Geometry: final body of the model. Coordinates: model frame, mm. A direction names the side the tool comes from. Coordinates: 2 decimals unless noted, no trailing zeros. Order: outer loops, then holes, each group sorted by start corner. A loop starts at its lowest first (then second) coordinate and runs counter-clockwise, first axis right, second up. Notation, with made-up numbers: M 60,71 L 69,71 A13 cw 69,82 Z; hole C -5,64.5 d9. An arc over 180 degrees is marked long. One line per question, with ' | ' between items.
from build123d import *

# Parameters (mm, degrees)
SKETCH1_W                    = 31.75
SKETCH1_H                    = 63.5
SKETCH1_W_2                  = 25.4
SKETCH1_H_2                  = 57.15
BOSS_EXTRUDE1_DEPTH          = 720.4964
CUT_EXTRUDE1_REACH           = 725.554
F_10_0_1935_DIAMETER_HOLE1_D = 4.9149
SKETCH3_R                    = 9.525
CUT_EXTRUDE2_DEPTH           = 3.175


with BuildPart() as part:
    # Sketch1 → Boss-Extrude1 (new body)
    with BuildSketch(Plane.XY):
        with Locations((3.710272719, -29.23968021)):
            Rectangle(SKETCH1_W, SKETCH1_H)
        with Locations((3.710272719, -29.23968021)):
            Rectangle(SKETCH1_W_2, SKETCH1_H_2, mode=Mode.SUBTRACT)
    extrude(amount=BOSS_EXTRUDE1_DEPTH)

    # Cut-Extrude1: up to this face of the body (flat: up to its plane)
    cut_extrude1_end = Plane(part.part.faces().sort_by_distance((3.710272719, -60.98968021, 360.2482))[0])
    # Sketch2 → Cut-Extrude1 (cut, up to the picked face)
    with BuildSketch(Plane(origin=(0, 2.51031979, 0), x_dir=(1, 0, 0), z_dir=(0, 1, 0)), mode=Mode.PRIVATE) as cut_extrude1_sk1:
        Polygon((-12.164727281, -31.75), (13.235272719, 0), (-12.164727281, 0), align=None)
    cut_extrude1_tool1 = split(extrude(cut_extrude1_sk1.sketch, amount=-CUT_EXTRUDE1_REACH, mode=Mode.PRIVATE), bisect_by=cut_extrude1_end, keep=Keep.BOTH, mode=Mode.PRIVATE)
    # Sketch2 → Cut-Extrude1 (cut, up to the picked face)
    with BuildSketch(Plane(origin=(0, 2.51031979, 0), x_dir=(1, 0, 0), z_dir=(0, 1, 0)), mode=Mode.PRIVATE) as cut_extrude1_sk2:
        Polygon((13.235272719, -720.4964), (-12.164727281, -688.7464), (-12.164727281, -720.4964), align=None)
    cut_extrude1_tool2 = split(extrude(cut_extrude1_sk2.sketch, amount=-CUT_EXTRUDE1_REACH, mode=Mode.PRIVATE), bisect_by=cut_extrude1_end, keep=Keep.BOTH, mode=Mode.PRIVATE)
    add(cut_extrude1_tool1.solids().sort_by(Axis((-3.698061, 2.51032, 10.583333), (0, -1, 0)))[0], mode=Mode.SUBTRACT)
    add(cut_extrude1_tool2.solids().sort_by(Axis((-3.698061, 2.51032, 709.913067), (0, -1, 0)))[0], mode=Mode.SUBTRACT)

    # #10 (0.1935) Diameter Hole1 (through all)
    with Locations(Plane(origin=(16.410272719, -10.18968021, 15.875), x_dir=(0, -1, 0), z_dir=(-1, 0, 0))):
        with Locations((0, 0), (38.1, 0), (0, 688.7464), (38.1, 688.7464)):
            Hole(F_10_0_1935_DIAMETER_HOLE1_D / 2)

    # Sketch3 → Cut-Extrude2 (cut)
    with BuildSketch(Plane.ZY.offset(-16.410272719)):
        with Locations(Location((15.875, -29.23968021, 0), (0, 0, 270))):
            Circle(SKETCH3_R)
        with Locations(Location((704.6214, -29.23968021, 0), (0, 0, 270))):
            Circle(SKETCH3_R)
    extrude(amount=-CUT_EXTRUDE2_DEPTH, mode=Mode.SUBTRACT)


solid = part.part
1. Section C-C, the plane x = 7.5. Output: boundary loops of the cut face in (y, z), and give its area (3 significant figures).
Response values:
outline: M -60.99,7.17 L -57.81,7.17 L -57.81,713.33 L -60.99,713.33 Z; M -0.66,7.17 L 2.51,7.17 L 2.51,713.33 L -0.66,713.33 Z | area: 4,480 mm^2
2. Draft query along Y for faces 3 (the face through (-9.87, -29.09, 28.88)), 4 (the face through (3, 2.51, 355)), 5 (the face through (17.976, -27.175, 695.323)). Return one class per face: pulls with the +Y half, pulls with the -Y half, needs draft (parallel to the pull), parting line crosses it, or undercut.
Response values:
face 3: needs draft | face 4: pulls with the +Y half | face 5: undercut
3. Pin query (flat end, axial travel): P1, Ø4, axis at y = -10.19, z = 704.62, coming from the -X side; P2, Ø8, axis at y = -10.19, z = 15.88, coming from the +X side; P3, Ø5.5, axis at y = -48.29, z = 704.62, coming from the -X side. Return the tip coordinate at first contact, or that it passes through.
Response values:
P1: passes through | P2: stops at x = 19.59 | P3: stops at x = 16.41
4. Section A-A, the plane z = 423. Output: boundary loops of the cut face in (x, y).
Response values:
outline: M -12.16,-60.99 L 19.59,-60.99 L 19.59,2.51 L -12.16,2.51 Z; hole M -8.99,-57.81 L 16.41,-57.81 L 16.41,-0.66 L -8.99,-0.66 Z
5. Material intervals for line 1 (X direction, y = -14.5, z = 176.5); line 2 (Y direction, x = -2.5, z = 656); line 3 (Z direction, x = -9.5, y = -53), sorted ascending. Write a range as [from, to].
Response values:
line 1: x = [-12.16, -8.99], [16.41, 19.59] | line 2: y = [-60.99, -57.81], [-0.66, 2.51] | line 3: z = [28.42, 692.08]
6. Section B-B, the plane y = -31.5. Output: boundary loops of the cut face in (x, z), and give its area (3 significant figures).
Response values:
outline: M -12.16,31.75 L -8.99,27.78 L -8.99,692.72 L -12.16,688.75 Z; M 16.41,0 L 19.59,0 L 19.59,6.62 L 16.41,6.62 Z; M 16.41,25.13 L 19.59,25.13 L 19.59,695.37 L 16.41,695.37 Z; M 16.41,713.87 L 19.59,713.87 L 19.59,720.5 L 16.41,720.5 Z | area: 4,270 mm^2
7. Access query for faces 1 (the face through (-9.754, -29.092, 691.76)), 2 (the face through (16.41, -30, 355)). Directions: +Z, -Z, +X, -X, +Y, -Y. A direction counts if a zero-diameter tool reaches every point of the face in a straight line with its end or side. Return the directions, or none.
Response values:
face 1: +Z, -X, +Y, -Y | face 2: +Z, -Z
